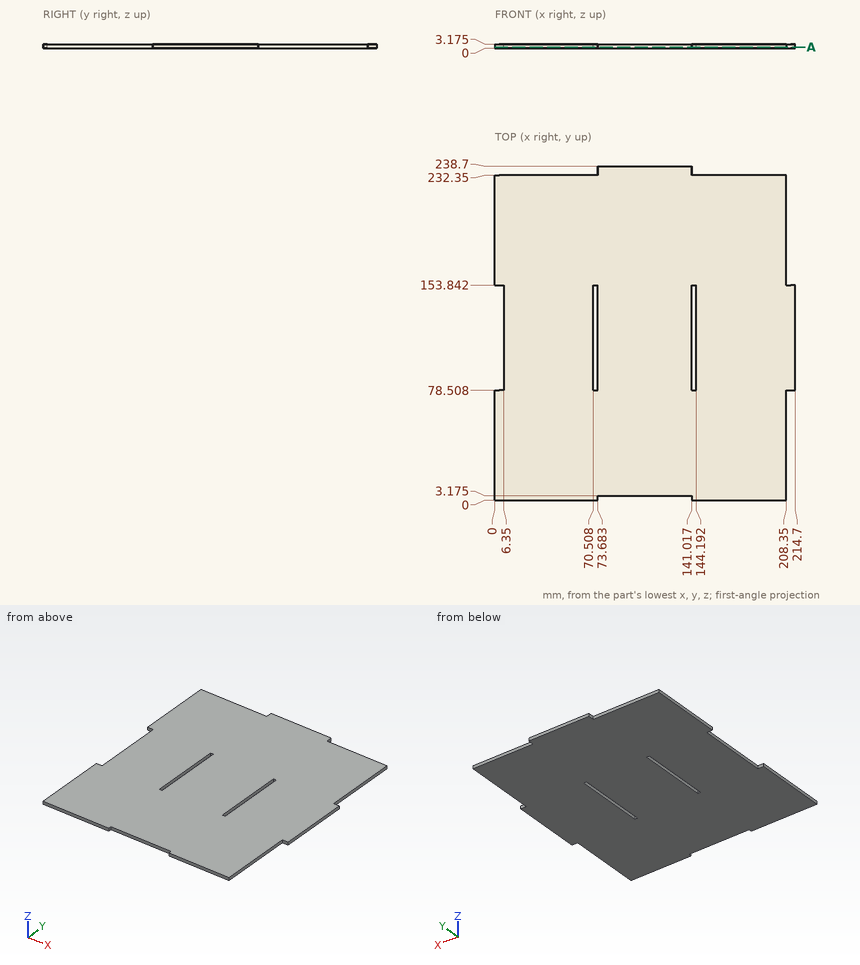
Check sheet for the drawn part. Datum: minimum x, y, z corner. Units: mm. Give positions to 0.01 mm unless a question says otherwise; leave off trailing zeros. Put each result on its own line as item: value.
1. Sectioned sample at A-A, the plane z = 1. Give the number of separate pieces and of enclosed holes in the cut face, plus the area to 3 significant figures.
Ans:
separate pieces: 1
enclosed holes: 2
area: 48,100 mm²
2. Thickness scan on line 1 (X direction, y = 141, z = 1.6); line 2 (Y direction, x = 118, z = 1.5) (1 decimal); line 3 (Y direction, x = 38.5, z = 1.75). Record the ranges inside material, lowest first.
Ans:
line 1: x = 6.35 to 70.51, 73.68 to 141.02, 144.19 to 214.7
line 2: y = 3.2 to 238.7
line 3: y = 0 to 232.35
3. Go/stop test with flat-tipped pins: pin 1 (1 mm diameter, centred on x = 73, z = 1.5, fed in from +Y); pin 2 (1 mm diameter, centred on x = 93, z = 1, fed in from -Y) (3 decimals); pin 3 (1 mm diameter, centred on x = 211, z = 2.5, fed in from -Y). Record where each tip stops, or that it passes through.
Ans:
pin 1: stops at y = 232.35
pin 2: stops at y = 3.175
pin 3: stops at y = 78.51
